Geometry: see drawing. Coordinates: mm, zero at the bounding-box minimum. A direction names the side the tool comes from. Give positions to 0.01 mm unless a question says otherwise; leave off trailing zeros. Write each loop counter-clockwise with the first axis right and the second up, starting at its lowest first coordinate (ties: lowest second). Pieces come first, ordered by that corner, then holes. Notation, with made-up numbers: (83.25, 6.25) - (113.25, 6.25) arc R11 ccw to (113.25, 20.25) - close; hole circle Ø4 at (78, 86). An arc over 180 degrees is marked (long way). Answer as CSV lines item,"result". Start each with the question number.
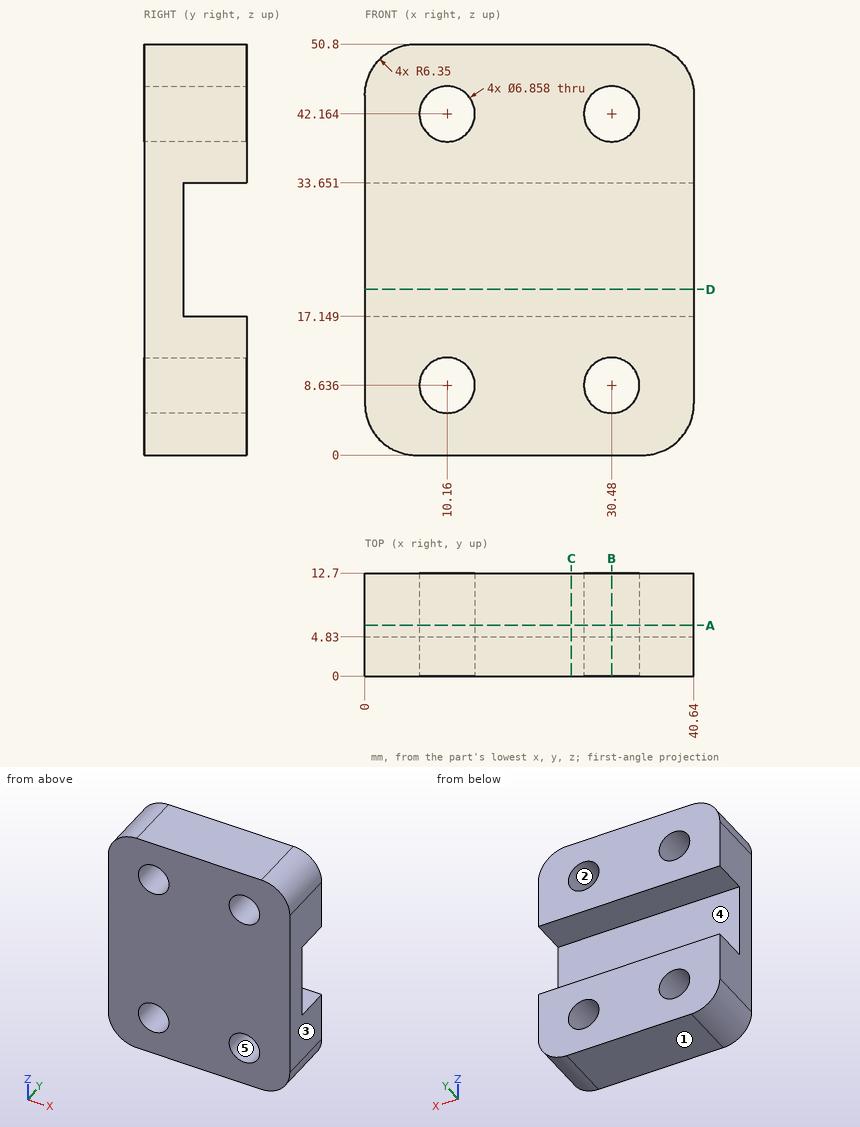
1) Material intervals for line 1 (Z direction, x = 11, y = 10.5); line 2 (Z direction, x = 8, y = 10.5); line 3 (X direction, y = 8.25, z = 41), sorted ascending. Write a range as from..to.
2) Contact query for flat-ended pins moving along their axis: P1, Ø3, axis at x = 23, y = 1.5, coming from the -Z side; P2, Ø5.5, axis at x = 10.16, z = 8.636, coming from the +Y side; P3, Ø5, axis at x = 19, z = 28, coming from the +Y side; P4, Ø1, axis at y = 5, z = 5.5, coming from the -X side. Output: stop coordinate, or through.
3) Cut plane B-B on x = 30.48. Output: boundary loops of the cut face in (y, z) (3 decimals), and give its area (3 significant figures).
4) Pull-direction query (Z, two-part tool) for the marked faces 1, 2 and 3; classes: +Z half, -Z half, draft (parallel to the pull), parting line (faces both ways), or undercut.
5) Reachability of the marked faces 4 and 5 from +Z, -Z, +X, -X, +Y, -Y: full face, straight path, thin tool, end or side. Return the list, or none.
6) Cut plane C-C on x = 25.5. Output: boundary loops of the cut face in (y, z).
7) Cut plane D-D on z = 20.5. Output: boundary loops of the cut face in (x, y), and give its area (3 significant figures).
8) Cut plane A-A on y = 6.25. Output: boundary loops of the cut face in (x, z) (3 decimals).
Numbers:
1,line 1,"z = 0..5.31, 11.96..17.15, 33.65..38.84, 45.49..50.8"
1,line 2,"z = 0..5.97, 11.3..17.15, 33.65..39.5, 44.83..50.8"
1,line 3,"x = 0..6.93, 13.39..27.25, 33.71..40.64"
2,P1,"stops at z = 0"
2,P2,"passes through"
2,P3,"stops at y = 4.83"
2,P4,"stops at x = 0.01"
3,outline,"(0, 0) - (12.7, 0) - (12.7, 5.207) - (0, 5.207) - close; (0, 12.065) - (12.7, 12.065) - (12.7, 17.149) - (4.83, 17.149) - (4.83, 33.651) - (12.7, 33.651) - (12.7, 38.735) - (0, 38.735) - close; (0, 45.593) - (12.7, 45.593) - (12.7, 50.8) - (0, 50.8) - close"
3,area,"341 mm²"
4,face 1,"-Z half"
4,face 2,"undercut"
4,face 3,"draft"
5,face 4,"+X, -X, +Y"
5,face 5,"+Y, -Y"
6,outline,"(0, 0) - (12.7, 0) - (12.7, 17.15) - (4.83, 17.15) - (4.83, 33.65) - (12.7, 33.65) - (12.7, 50.8) - (0, 50.8) - close"
7,outline,"(0, 0) - (40.64, 0) - (40.64, 4.83) - (0, 4.83) - close"
7,area,"196 mm²"
8,outline,"(0, 6.35) arc R6.35 ccw to (6.35, 0) - (34.29, 0) arc R6.35 ccw to (40.64, 6.35) - (40.64, 17.149) - (0, 17.149) - close; (0, 33.651) - (40.64, 33.651) - (40.64, 44.45) arc R6.35 ccw to (34.29, 50.8) - (6.35, 50.8) arc R6.35 ccw to (0, 44.45) - close; hole circle Ø6.858 at (10.16, 8.636); hole circle Ø6.858 at (10.16, 42.164); hole circle Ø6.858 at (30.48, 8.636); hole circle Ø6.858 at (30.48, 42.164)"
